Check sheet for the modelled part. Datum: model origin and axes. Units: mm. A direction names the side the tool comes from. Round coordinates to 2 decimals unless told otherwise and drop trailing zeros. Loops run counter-clockwise (first coordinate to the right, second up) from the corner with the lowest first, then second, coordinate; pieces in that order, holes last. Notation, with made-up numbers: (13, 85) -> (71, 85) arc R20 ccw to (71, 99) -> close; hole circle Ø4 at (-11.75, 78.5). An arc over 180 degrees is marked (long way). Use one line per item in the form item = value. Start each with the question number.
(1) Draft check along Y on faces 4 (the cylindrical face through (0.6, 0.57, 11.15)), 5 (the flat face through (17, 13, 1)), 6 (the cylindrical face through (0.57, 29.4, 11.15)). Enter one of: released by +Y, released by -Y, zero draft, split by the parting line, or undercut.
(2) Sectioned sample at D-D (x = 28). Record the cut outline in (y, z).
(3) Sectioned sample at C-C (y = 12). Record the cut outline in (x, z), and give its area (3 significant figures).
(4) Go/stop test with flat-tipped pins: pin 1 (10 mm diameter, centred on x = 48, y = 14, fed in from +Z); pin 2 (3 mm diameter, centred on x = 26.5, y = 12, fed in from -Z). Record where each tip stops, or that it passes through.
(5) Material ranges on probe 1 along X at (y, z) = (6.75, 4.25); probe 2 along Y at (x, z) = (9, 20.75); probe 3 along Z at (x, y) = (66, 21), recorded low to high. Write a range as [from, to].
(6) Sectioned sample at A-A (x = 56). Record the cut outline in (y, z).
(7) Sectioned sample at B-B (z = 11.5). Record the cut outline in (x, y).
(8) Set-up check for faces 1 (the flat face through (32.2, 1.7, 22)), 2 (the flat face through (35, 2, 12)), 3 (the cylindrical face through (8, 15, 1)): record each of +Z, -Z, +X, -X, +Y, -Y from which the full face is reachable in a straight line by a thin tool's end or side.
from build123d import *

# Parameters (mm, degrees)
CROQUIS1_W              = 70
CROQUIS1_H              = 30
SALIENTE_EXTRUIR4_DEPTH = 22
CROQUIS5_W              = 66
CROQUIS5_H              = 26
CORTAR_EXTRUIR1_DEPTH   = 20
CORTAR_EXTRUIR3_DEPTH   = 20
REDONDEO2_R             = 2
REDONDEO3_R             = 2
REDONDEO4_R             = 2
REDONDEO5_R             = 2


with BuildPart() as part:
    # Croquis1 → Saliente-Extruir4 (new body)
    with BuildSketch(Plane.XY):
        with Locations((35, 15)):
            Rectangle(CROQUIS1_W, CROQUIS1_H)
    extrude(amount=SALIENTE_EXTRUIR4_DEPTH)

    # Croquis5 → Cortar-Extruir1 (cut)
    with BuildSketch(Plane.XY.offset(22)):
        with Locations((35, 15)):
            Rectangle(CROQUIS5_W, CROQUIS5_H)
    extrude(amount=-CORTAR_EXTRUIR1_DEPTH, mode=Mode.SUBTRACT)

    # Croquis6 → Cortar-Extruir3 (cut)
    with BuildSketch(Plane.XY.offset(2)):
        with BuildLine():
            Line((10, 17), (24, 17))
            ThreePointArc((24, 17), (26, 15), (24, 13))
            Line((24, 13), (10, 13))
            ThreePointArc((10, 13), (8, 15), (10, 17))
        make_face()
        with BuildLine():
            Line((60, 17), (46, 17))
            ThreePointArc((46, 17), (44, 15), (46, 13))
            Line((46, 13), (60, 13))
            ThreePointArc((60, 13), (62, 15), (60, 17))
        make_face()
    extrude(amount=-CORTAR_EXTRUIR3_DEPTH, mode=Mode.SUBTRACT)

    # Redondeo2
    redondeo2_edges = [part.edges().sort_by_distance(p)[0] for p in [
        (70, 0, 11),
    ]]
    fillet(redondeo2_edges, radius=REDONDEO2_R)

    # Redondeo3
    redondeo3_edges = [part.edges().sort_by_distance(p)[0] for p in [
        (70, 30, 11),
    ]]
    fillet(redondeo3_edges, radius=REDONDEO3_R)

    # Redondeo4
    redondeo4_edges = [part.edges().sort_by_distance(p)[0] for p in [
        (0, 0, 11),
    ]]
    fillet(redondeo4_edges, radius=REDONDEO4_R)

    # Redondeo5
    redondeo5_edges = [part.edges().sort_by_distance(p)[0] for p in [
        (0, 30, 11),
    ]]
    fillet(redondeo5_edges, radius=REDONDEO5_R)


solid = part.part
Checks:
q1.face_4 = released by -Y
q1.face_5 = undercut
q1.face_6 = released by +Y
q2.outline = (0, 0) -> (30, 0) -> (30, 22) -> (28, 22) -> (28, 2) -> (2, 2) -> (2, 22) -> (0, 22) -> close
q3.outline = (0, 0) -> (70, 0) -> (70, 22) -> (68, 22) -> (68, 2) -> (2, 2) -> (2, 22) -> (0, 22) -> close
q3.area = 220 mm2
q4.pin_1 = 2
q4.pin_2 = 0
q5.probe_1 = [0, 2], [68, 70]
q5.probe_2 = [0, 2], [28, 30]
q5.probe_3 = [0, 2]
q6.outline = (0, 0) -> (13, 0) -> (13, 2) -> (2, 2) -> (2, 22) -> (0, 22) -> close; (17, 0) -> (30, 0) -> (30, 22) -> (28, 22) -> (28, 2) -> (17, 2) -> close
q7.outline = (0, 2) arc R2 ccw to (2, 0) -> (68, 0) arc R2 ccw to (70, 2) -> (70, 28) arc R2 ccw to (68, 30) -> (2, 30) arc R2 ccw to (0, 28) -> close; hole (2, 2) -> (68, 2) -> (68, 28) -> (2, 28) -> close
q8.face_1 = +Z, +X, -X, +Y, -Y
q8.face_2 = +Z
q8.face_3 = +Z, -Z
